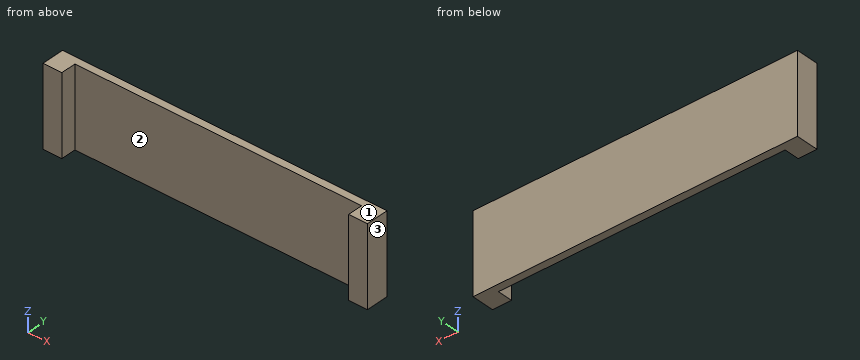
```python
from build123d import *

# Parameters (mm, degrees)
SKETCH1_W                       = 860
SKETCH1_H                       = 210
BOSS_EXTRUDE1_DEPTH             = 20
BOSS_EXTRUDE2_REACH             = 445.086
SKETCH2_W                       = 50
SKETCH2_H                       = 40
BOSS_EXTRUDE2_DIRECTION_2_REACH = 445.086


with BuildPart() as part:
    # Sketch1 → Boss-Extrude1 (new body)
    with BuildSketch(Plane(origin=(0, 0, 0), x_dir=(1, 0, 0), z_dir=(0, 1, 0))):
        Rectangle(SKETCH1_W, SKETCH1_H)
    extrude(amount=BOSS_EXTRUDE1_DEPTH)

    # Boss-Extrude2: up to this face of the body (flat: up to its plane)
    boss_extrude2_end = Plane(part.part.faces().sort_by_distance((0, 10, 105))[0])
    # Sketch2 → Boss-Extrude2 (add, up to the picked face)
    with BuildSketch(Plane.XY, mode=Mode.PRIVATE) as boss_extrude2_sk1:
        with Locations((-405, -20)):
            Rectangle(SKETCH2_W, SKETCH2_H)
    boss_extrude2_tool1 = split(extrude(boss_extrude2_sk1.sketch, amount=BOSS_EXTRUDE2_REACH, mode=Mode.PRIVATE), bisect_by=boss_extrude2_end, keep=Keep.BOTH, mode=Mode.PRIVATE)
    # Sketch2 → Boss-Extrude2 (add, up to the picked face)
    with BuildSketch(Plane.XY, mode=Mode.PRIVATE) as boss_extrude2_sk2:
        with Locations((405, -20)):
            Rectangle(SKETCH2_W, SKETCH2_H)
    boss_extrude2_tool2 = split(extrude(boss_extrude2_sk2.sketch, amount=BOSS_EXTRUDE2_REACH, mode=Mode.PRIVATE), bisect_by=boss_extrude2_end, keep=Keep.BOTH, mode=Mode.PRIVATE)
    add(boss_extrude2_tool1.solids().sort_by(Axis((-405, -20, 0), (0, 0, 1)))[0])
    add(boss_extrude2_tool2.solids().sort_by(Axis((405, -20, 0), (0, 0, 1)))[0])

    # Boss-Extrude2 direction 2: up to this face of the body (flat: up to its plane)
    boss_extrude2_direction_2_end = Plane(part.part.faces().sort_by_distance((0, 10, -105))[0])
    # Sketch2 → Boss-Extrude2 direction 2 (add, up to the picked face)
    with BuildSketch(Plane.XY, mode=Mode.PRIVATE) as boss_extrude2_direction_2_sk1:
        with Locations((-405, -20)):
            Rectangle(SKETCH2_W, SKETCH2_H)
    boss_extrude2_direction_2_tool1 = split(extrude(boss_extrude2_direction_2_sk1.sketch, amount=-BOSS_EXTRUDE2_DIRECTION_2_REACH, mode=Mode.PRIVATE), bisect_by=boss_extrude2_direction_2_end, keep=Keep.BOTH, mode=Mode.PRIVATE)
    # Sketch2 → Boss-Extrude2 direction 2 (add, up to the picked face)
    with BuildSketch(Plane.XY, mode=Mode.PRIVATE) as boss_extrude2_direction_2_sk2:
        with Locations((405, -20)):
            Rectangle(SKETCH2_W, SKETCH2_H)
    boss_extrude2_direction_2_tool2 = split(extrude(boss_extrude2_direction_2_sk2.sketch, amount=-BOSS_EXTRUDE2_DIRECTION_2_REACH, mode=Mode.PRIVATE), bisect_by=boss_extrude2_direction_2_end, keep=Keep.BOTH, mode=Mode.PRIVATE)
    add(boss_extrude2_direction_2_tool1.solids().sort_by(Axis((-405, -20, 0), (0, 0, -1)))[0])
    add(boss_extrude2_direction_2_tool2.solids().sort_by(Axis((405, -20, 0), (0, 0, -1)))[0])


solid = part.part
```
Can you work these out from the model? Positions are in its coordinate system, mm. Face numbers are marked on the shaded views. Coordinates: 2 decimals unless noted, no trailing zeros. Loops run counter-clockwise (first coordinate to the right, second up) from the corner with the lowest first, then second, coordinate; pieces in that order, holes last. Notation, with made-up numbers: (-36.5, -8) - (-14.5, -8) arc R20 cw to (-14.5, 19) - close; hole circle Ø4 at (61.5, 6.25). An arc over 180 degrees is marked (long way). Answer as CSV lines item,"result". Start each with the question number.
1) Thinking about a two-plate mould opening in X: for the marked faces 1, 2 and 3, which applies, pulls with the +X half, pulls with the -X half, needs draft (parallel to the pull), parting line crosses it, or undercut?
2) For pin 1 (12 mm diameter, centred on x = 268, y = -3, fed in from -Z), with a flat end and sliding along its axis, tell me the tip position at first contact or that it passes through.
3) Suppose I cut it at B-B (z = 0.5). Please give me the cut outline in (x, y), plus the area to 3 significant figures.
4) I need wall thicknesses on line 1 (X direction, y = -30.5, z = -52.5); line 2 (Y direction, x = -110.5, z = -57.5). Which ranges of each line are inside material? Lowest first, please. Write a range as from..to.
5) Suppose I cut it at C-C (x = 318). Please give me the cut outline in (y, z), plus the area to 3 significant figures.
6) Suppose I cut it at A-A (y = -15). Please give me the cut outline in (x, z), plus the area to 3 significant figures.
Check result:
1,face 1,"needs draft"
1,face 2,"undercut"
1,face 3,"pulls with the +X half"
2,pin 1,"stops at z = -105"
3,outline,"(-430, -40) - (-380, -40) - (-380, 0) - (380, 0) - (380, -40) - (430, -40) - (430, 20) - (-430, 20) - close"
3,area,"21,200 mm²"
4,line 1,"x = -430..-380, 380..430"
4,line 2,"y = 0..20"
5,outline,"(0, -105) - (20, -105) - (20, 105) - (0, 105) - close"
5,area,"4,200 mm²"
6,outline,"(-430, -105) - (-380, -105) - (-380, 105) - (-430, 105) - close; (380, -105) - (430, -105) - (430, 105) - (380, 105) - close"
6,area,"21,000 mm²"
